Source: CAD feature listing. Evaluate the final solid. Frame: model axes, mm. Coordinates: 2 decimals unless noted, no trailing zeros. Write each loop counter-clockwise with the first axis right and the second up, starting at its lowest first coordinate (ties: lowest second). Pieces come first, ordered by that corner, then holes. Notation, with made-up numbers: M 71.5,53 L 89.5,53 A17 ccw 89.5,79 Z; hole C 38.25,27.25 d6. An arc over 180 degrees is marked long. One line per item, written item: value. Start each with the question number.
Item 1: Ray query, L1, parallel to Y at x = 1.25, z = 558; L2, parallel to X at y = -6.5, z = 242; L3, parallel to X at y = 15, z = 114. Return the intervals inside material, ascending. Write a range as from..to.
Item 2: Cut plane B-B, the plane y = -23. Output: boundary loops of the cut face in (x, z), then the cut area to 3 significant figures.
Item 3: Pin query (flat end, axial travel): P1, Ø2, axis at x = -8.5, y = 7, coming from the +Z side. Return the tip coordinate at first contact, or that it passes through.
Item 4: Cut plane A-A, the plane x = -6.5. Output: boundary loops of the cut face in (y, z), then the cut area to 3 significant figures.
Item 5: Cut plane C-C, the plane z = 358.5. Output: boundary loops of the cut face in (x, y), then the cut area to 3 significant figures.
Autodesk Inventor part; units mm, degrees
ref_plane "YZ Plane" through (0, 0, 0) normal (1, 0, 0) x (0, 1, 0)
ref_plane "XZ Plane" through (0, 0, 0) normal (0, 1, 0) x (-1, 0, 0)
ref_plane "XY Plane" through (0, 0, 0) normal (0, 0, 1) x (1, 0, 0)
sketch "Sketch1" plane through (0, 0, 0) normal (0, 0, 1) x (1, 0, 0)
  line L0 (-12.1708, 16.0073) -> (13.2292, 16.0073)
  line L1 (13.2292, 16.0073) -> (13.2292, -34.7927)
  line L2 (13.2292, -34.7927) -> (-12.1708, -34.7927)
  line L3 (-12.1708, -34.7927) -> (-12.1708, 16.0073)
  line L4 (11.9592, 14.7373) -> (-10.9008, 14.7373)
  line L5 (-10.9008, 14.7373) -> (-10.9008, -33.5227)
  line L6 (-10.9008, -33.5227) -> (11.9592, -33.5227)
  line L7 (11.9592, -33.5227) -> (11.9592, 14.7373)
  point P0 (0, 0)
  dimension "d0" = 25.4
  dimension "d1" = 50.8
  dimension "d2" = 1.27
extrude "Extrusion1" add sketch "Sketch1" along normal blind 762
sketch "Sketch2" plane through (-12.1708, 16.0073, 0) normal (0, 1, 0) x (1, 0, 0)
  circle A0 centre (12.7, -12.7) radius 1.7272
  line L0 (25.4, 0) -> (0, 0)
  line L1 (0, 0) -> (0, -762)
  point P0 (12.1708, 0)
  dimension "d5" = 3.4544
  dimension "d6" = 12.7
  dimension "d7" = 12.7
extrude "Extrusion2" cut sketch "Sketch2" against normal through all
pattern_linear "Rectangular Pattern1" count 30 spacing 25.4 along (0, 0, 1) of "Extrusion2"
sketch "Sketch3" plane through (-12.1708, 16.0073, 0) normal (0, 1, 0) x (1, 0, 0)
  line L0 (0, 0) -> (25.4, 0)
  line L1 (25.4, 0) -> (25.4, -50.8)
  line L2 (25.4, -50.8) -> (0, -50.8)
  line L3 (0, -50.8) -> (0, 0)
  line L4 (25.4, 0) -> (0, 0)
  line L5 (0, 0) -> (0, -762)
  point P0 (12.1708, 0)
  dimension "d13" = 25.4
  dimension "d14" = 50.8
extrude "Extrusion3" cut sketch "Sketch3" against normal through all
properties part number "VerseFrame 28in"
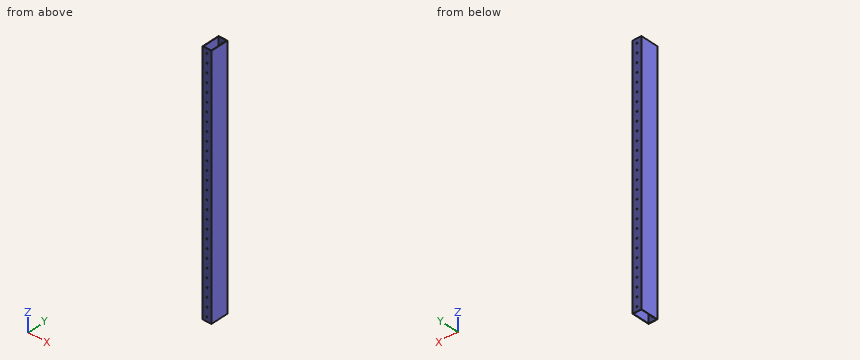
From the geometry:
1. L1: y = -34.79..-33.52, 14.74..16.01
1. L2: x = -12.17..-10.9, 11.96..13.23
1. L3: x = -12.17..-1.17, 2.23..13.23
2. outline: M -12.17,50.8 L -10.9,50.8 L -10.9,762 L -12.17,762 Z; M 11.96,50.8 L 13.23,50.8 L 13.23,762 L 11.96,762 Z
2. area: 1,810 mm²
3. P1: passes through
4. outline: M -34.79,50.8 L -33.52,50.8 L -33.52,762 L -34.79,762 Z; M 14.74,50.8 L 16.01,50.8 L 16.01,762 L 14.74,762 Z
4. area: 1,810 mm²
5. outline: M -12.17,-34.79 L 13.23,-34.79 L 13.23,16.01 L -12.17,16.01 Z; hole M -10.9,-33.52 L 11.96,-33.52 L 11.96,14.74 L -10.9,14.74 Z
5. area: 187 mm²
